```python
from build123d import *

# Parameters (mm, degrees)
BOSS_EXTRUDE1_OUTLINE_W        = 127.25
BOSS_EXTRUDE1_OUTLINE_H        = 35
BOSS_EXTRUDE1_OUTLINE_R        = 2.38125
BOSS_EXTRUDE1_DEPTH            = 10
BOSS_EXTRUDE2_DEPTH            = 70
BOSS_EXTRUDE2_DEPTH_BACK       = 50
SKETCH2_W                      = 10
SKETCH2_H                      = 35
CHAMFER1_SIZE                  = 10
SKETCH8_W                      = 35
SKETCH8_H                      = 5
BOSS_EXTRUDE4_DEPTH            = 40
SKETCH9_W                      = 35
SKETCH9_H                      = 23.5
BOSS_EXTRUDE5_DEPTH            = 5
M8_CLEARANCE_HOLE2_D           = 9
M8_CLEARANCE_HOLE2_DEPTH       = 23
M8_CLEARANCE_HOLE2_CSINK_D     = 9.05
M8_CLEARANCE_HOLE2_CSINK_ANGLE = 90
M8_CLEARANCE_HOLE2_TIP         = 2.703872786


# Read off the part's stored shape, not the designer's step: Boss-Extrude1
with BuildPart() as part:
    # Boss-Extrude1 outline → Boss-Extrude1 (new body)
    with BuildSketch(Plane(origin=(0, 0, 0), x_dir=(1, 0, 0), z_dir=(0, 1, 0))):
        with Locations((-38.225, 0)):
            Rectangle(BOSS_EXTRUDE1_OUTLINE_W, BOSS_EXTRUDE1_OUTLINE_H)
        with Locations((-19.85, -10.3252)):
            Circle(BOSS_EXTRUDE1_OUTLINE_R, mode=Mode.SUBTRACT)
        with Locations((19.8502, -10.3252)):
            Circle(BOSS_EXTRUDE1_OUTLINE_R, mode=Mode.SUBTRACT)
        with Locations((-19.85, 10.325)):
            Circle(BOSS_EXTRUDE1_OUTLINE_R, mode=Mode.SUBTRACT)
        with Locations((19.8502, 10.325)):
            Circle(BOSS_EXTRUDE1_OUTLINE_R, mode=Mode.SUBTRACT)
    extrude(amount=BOSS_EXTRUDE1_DEPTH)

    # Sketch2 → Boss-Extrude2 (add, two sides: drawn at the far end of the back side and taken through both)
    with BuildSketch(Plane(origin=(0, 10, 0), x_dir=(1, 0, 0), z_dir=(0, 1, 0)).offset(-BOSS_EXTRUDE2_DEPTH_BACK)):
        with Locations((-56.85, 0)):
            Rectangle(SKETCH2_W, SKETCH2_H)
    extrude(amount=BOSS_EXTRUDE2_DEPTH + BOSS_EXTRUDE2_DEPTH_BACK)

    # Chamfer1
    chamfer1_edges = [part.edges().sort_by_distance(p)[0] for p in [
        (-51.85, -40, 0),
    ]]
    chamfer(chamfer1_edges, length=CHAMFER1_SIZE - 0.0001)  # a hair under: the kernel refuses the full size

    # Sketch8 → Boss-Extrude4 (add)
    with BuildSketch(Plane.ZY.offset(61.85)):
        with Locations((0, 36)):
            Rectangle(SKETCH8_W, SKETCH8_H)
    extrude(amount=BOSS_EXTRUDE4_DEPTH)

    # Sketch9 → Boss-Extrude5 (add)
    with BuildSketch(Plane.ZY.offset(101.85)):
        with Locations((0, 21.75)):
            Rectangle(SKETCH9_W, SKETCH9_H)
    extrude(amount=-BOSS_EXTRUDE5_DEPTH)

    # M8 Clearance Hole2
    with Locations(Plane(origin=(-51.85, 0, 0), x_dir=(0, 0, -1), z_dir=(1, 0, 0))):
        with Locations((0, 60), (0, -20)):
            CounterSinkHole(M8_CLEARANCE_HOLE2_D / 2, M8_CLEARANCE_HOLE2_CSINK_D / 2, depth=M8_CLEARANCE_HOLE2_DEPTH, counter_sink_angle=M8_CLEARANCE_HOLE2_CSINK_ANGLE)
            with Locations((0, 0, -(M8_CLEARANCE_HOLE2_DEPTH + M8_CLEARANCE_HOLE2_TIP / 2))):  # 118° drill point
                Cone(0, M8_CLEARANCE_HOLE2_D / 2, M8_CLEARANCE_HOLE2_TIP, mode=Mode.SUBTRACT)


solid = part.part
```
Geometry: final body of the model. Coordinates: model frame, mm. A direction names the side the tool comes from. Coordinates: 2 decimals unless noted, no trailing zeros. Order: outer loops, then holes, each group sorted by start corner. A loop starts at its lowest first (then second) coordinate and runs counter-clockwise, first axis right, second up. Notation, with made-up numbers: (64, 88) - (94, 88) arc R34 ccw to (94, 123) - close; hole circle Ø7 at (-40, 40). An arc over 180 degrees is marked (long way). Return JSON: item names as keys, results as strings. Group by question number.
1. Set-up query: faces 1 (the face through (-14, 0, 0)), 2 (the face through (-56.93, -15.54, -0.59)), 3 (the face through (-80, 10, 0)), 4 (the face through (-61.85, 54, 0)). Return all of +Z, -Z, +X, -X, +Y, -Y with unobstructed straight access to the full face (end or side cutting, diameter ignored); none if empty.
2. Cut plane D-D (y = -20). Output: boundary loops of the cut face in (x, z) (3 decimals).
3. Pull-direction query (X, two-part tool) for faces 5 (the face through (-18.751, 4.93, 12.438)), 6 (the face through (-51.85, -15, 0)), 7 (the face through (-53, 15, -17.5)); classes: pulls with the +X half, pulls with the -X half, needs draft (parallel to the pull), parting line crosses it, or undercut.
4. Cut plane C-C (y = 25). Output: boundary loops of the cut face in (x, z).
5. Pin query (flat end, axial travel): pin 1 (5 mm diameter, centred on y = -25.5, z = -11.5, fed in from -X); pin 2 (3 mm diameter, centred on x = 19.85, z = 10.33, fed in from +Y); pin 3 (1.5 mm diameter, centred on x = -85, z = -3, fed in from -Y); pin 4 (7.5 mm diameter, centred on x = -19.85, z = -10.325, fed in from +Y). Return the tip coordinate at first contact, or that it passes through.
6. Material intervals for line 1 along X through (y, z) = (32, -8.5); line 2 along Y through (x, z) = (-67.5, 12.5); line 3 along Z through (x, y) = (-58, -20), sorted ascending. Write a range as [from, to].
7. Cut plane B-B (x = -66.5). Output: boundary loops of the cut face in (y, z).
8. Cut plane A-A (z = 0). Count the separate pieces of the cut face and the enclosed holes in it, plus the area to 3 significant figures.
Resolved:
{
 "1": {"face 1": "+Z, -Z, +X, -Y", "face 2": "+X, -X", "face 3": "+Z, -Z", "face 4": "+Z, -Z, -X, +Y"},
 "2": {"outline": "(-61.85, -17.5) - (-51.85, -17.5) - (-51.85, -4.525) - (-51.875, -4.5) - (-61.85, -4.5) - close; (-61.85, 4.5) - (-51.875, 4.5) - (-51.85, 4.525) - (-51.85, 17.5) - (-61.85, 17.5) - close"},
 "3": {"face 5": "undercut", "face 6": "pulls with the +X half", "face 7": "needs draft"},
 "4": {"outline": "(-101.85, -17.5) - (-96.85, -17.5) - (-96.85, 17.5) - (-101.85, 17.5) - close; (-61.85, -17.5) - (-51.85, -17.5) - (-51.85, 17.5) - (-61.85, 17.5) - close"},
 "5": {"pin 1": "stops at x = -61.85", "pin 2": "passes through", "pin 3": "stops at y = 0", "pin 4": "stops at y = 10"},
 "6": {"line 1": "x = [-101.85, -96.85], [-61.85, -51.85]", "line 2": "y = [0, 10], [33.5, 38.5]", "line 3": "z = [-17.5, -4.5], [4.5, 17.5]"},
 "7": {"outline": "(0, -17.5) - (10, -17.5) - (10, 17.5) - (0, 17.5) - close; (33.5, -17.5) - (38.5, -17.5) - (38.5, 17.5) - (33.5, 17.5) - close"},
 "8": {"separate pieces": "3", "enclosed holes": "1", "area": "2,460 mm²"}
}
